Work out the finished part from the listing and answer in its coordinate system (mm). A direction names the side the tool comes from. Coordinates: 2 decimals unless noted, no trailing zeros. Order: outer loops, then holes, each group sorted by start corner. A loop starts at its lowest first (then second) coordinate and runs counter-clockwise, first axis right, second up. Notation, with made-up numbers: (4, -11.75) - (55, -11.75) arc R12 ccw to (55, -4.75) - close; hole circle Ø10 at (-6.5, 50.25). An arc over 180 degrees is marked (long way). Answer as a JSON object with one key per item and string values. Group by question number.
1) The mould has two halves that part along Z. Classify faces 1 (the face through (0, 10, -38.1)), 2 (the face through (12, 0, 9)), 3 (the face through (15.19, 19.19, -3.37)), 4 (the face through (-16.59, 10.14, 37.15)): released by +Z, released by -Z, zero draft, split by the parting line, or undercut.
2) Find the intervals of material crossed by line 1 along X through (y, z) = (6.5, 0); line 2 along X through (y, z) = (19.3, 0); line 3 along Y through (x, z) = (14.5, -0.5), in increasing order.
3) Section A-A (x = 0) is taken. Give the vertices of the cut face in (y, z), plus the area to 3 significant figures.
4) Section C-C (z = 0) is taken. Give the vertices of the cut face in (x, y), plus the area to 3 significant figures.
5) A tool of negligible diameter and unlimited length cuts with its end or side. For faces 5 (the face through (13, 18.412, 7)), 6 (the face through (-16.55, 10.14, -37.19)), from which of +Z, -Z, +X, -X, +Y, -Y can it reach the whole face along a straight path? Write none if from no direction.
Autodesk Inventor part; units mm, degrees
ref_plane "YZ Plane" through (0, 0, 0) normal (1, 0, 0) x (0, 1, 0)
ref_plane "XZ Plane" through (0, 0, 0) normal (0, 1, 0) x (-1, 0, 0)
ref_plane "XY Plane" through (0, 0, 0) normal (0, 0, 1) x (1, 0, 0)
sketch "Sketch1" plane through (0, 0, 0) normal (0, 1, 0) x (-1, 0, 0)
  line L0 (0, -53.34) -> (0, 53.34)
  line L1 (-24.5, 0) -> (24.5, 0)
  line L2 (24.5, 0) -> (-24.5, 0)
  line L3 (0, -53.34) -> (0, 53.34)
  line L4 (-17.5, 38.1) -> (-17.5, -38.1)
  line L5 (-17.5, -38.1) -> (17.5, -38.1)
  line L6 (17.5, -38.1) -> (17.5, 38.1)
  line L7 (17.5, 38.1) -> (-17.5, 38.1)
  line L8 (-17.5, -38.1) -> (17.5, 38.1) construction
  point P0 (0, 0)
  dimension "d1" = 76.2
  dimension "d2" = 35
extrude "Extrusion1" add sketch "Sketch1" along normal blind 20
sketch "Sketch2" plane through (0, 20, 0) normal (0, 1, 0) x (1, 0, 0)
  point P0 (0, 0)
  point P1 (0, 0)
hole "Hole1" at (0, 20, 0) direction (0, -1, 0) diameter 28.575 end through all counterbore diameter 31.12 counterbore depth 1.588
fillet "Fillet1" radius 3.175 4 edges at (17.5, 10, 38.1) (17.5, 10, -38.1) (-17.5, 10, 38.1) (-17.5, 10, -38.1)
properties part number "BearingBlock"
Report:
{
 "1": {"face 1": "released by -Z", "face 2": "zero draft", "face 3": "undercut", "face 4": "released by +Z"},
 "2": {"line 1": "x = -17.5 to -14.29, 14.29 to 17.5", "line 2": "x = -17.5 to -15.56, 15.56 to 17.5", "line 3": "y = 0 to 18.41"},
 "3": {"outline": "(0, -38.1) - (20, -38.1) - (20, -15.56) - (18.41, -15.56) - (18.41, -14.29) - (0, -14.29) - close; (0, 14.29) - (18.41, 14.29) - (18.41, 15.56) - (20, 15.56) - (20, 38.1) - (0, 38.1) - close", "area": "948 mm²"},
 "4": {"outline": "(-17.5, 0) - (-14.29, 0) - (-14.29, 18.41) - (-15.56, 18.41) - (-15.56, 20) - (-17.5, 20) - close; (14.29, 0) - (17.5, 0) - (17.5, 20) - (15.56, 20) - (15.56, 18.41) - (14.29, 18.41) - close", "area": "124 mm²"},
 "5": {"face 5": "+Y", "face 6": "-Z, -X, +Y, -Y"}
}
